Design review of the part built by this model. Coordinates are the model's own, in mm. Face numbers are marked on the shaded views. A direction names the side the tool comes from. Coordinates: 2 decimals unless noted, no trailing zeros. Loops run counter-clockwise (first coordinate to the right, second up) from the corner with the lowest first, then second, coordinate; pieces in that order, holes last. Notation, with made-up numbers: M 69.25,-34.75 L 101.25,-34.75 A23 cw 101.25,-22.75 Z; hole C 36.25,-10.5 d9. An arc over 180 degrees is marked long. Answer as a JSON object with one key per item and string values. Group by question number.
1. Consider section C-C (z = 48.5). State the section outline as (x, y) points.
2. Draft analysis for pull direction X (two halves, no side actions). For the marked faces 4, 5 and 6, state which applies: +X half, -X half, draft (parallel to the pull), parting line (faces both ways), or undercut.
3. Insertion check: pin 1 (1.8 mm diameter, centred on x = 4.22, z = -16.15, fed in from -Y); pin 2 (12 mm diameter, centred on x = 3.5, z = -18.5, fed in from -Y); pin 3 (0.6 mm diameter, centred on y = 1, z = 9, fed in from -X); pin 4 (1 mm diameter, centred on y = 1, z = -19, fed in from +X). Each pin has a flat end and moves straight along its axis. Give the tip position at first contact, or say it passes through.
4. To check wall thickness, follow probe 1 along X at (y, z) = (-17, 42); probe 2 along Y at (x, z) = (22.5, 45.5); probe 3 along Z at (x, y) = (16, -32). State the ranges of each line that lie inside material, in increasing order.
5. Machinability: for the marked faces 1, 2 and 3, which of the approach directions +Z, -Z, +X, -X, +Y, -Y give a long, thin tool a straight path to every point of the face, cutting with its end or side? Answer none if there is none.
6. Consider section A-A (x = -10). State the section outline as (y, z) points, then the cut area to 3 significant figures.
7. Consider section B-B (y = -3). State the section outline as (x, z) points, then the cut area to 3 significant figures.
8. Consider section D-D (z = -1). State the section outline as (x, y) points.
from build123d import *

# Parameters (mm, degrees)
BOSS_EXTRUDE1_DEPTH = 2
SKETCH3_W           = 60.33
SKETCH3_H           = 20
BOSS_EXTRUDE2_DEPTH = 30
SKETCH4_W           = 54.33
SKETCH4_H           = 27
CUT_EXTRUDE1_DEPTH  = 20
SKETCH5_R           = 1.5
CUT_EXTRUDE2_DEPTH  = 2
SKETCH6_W           = 60.33
SKETCH6_H           = 20
BOSS_EXTRUDE3_DEPTH = 5
SKETCH8_W           = 54.33
SKETCH8_H           = 20
CUT_EXTRUDE3_DEPTH  = 3
SKETCH9_W           = 24.33
SKETCH9_H           = 20
BOSS_EXTRUDE4_DEPTH = 2
SKETCH10_R          = 2.5
CUT_EXTRUDE4_DEPTH  = 2


with BuildPart() as part:
    # Sketch2 → Boss-Extrude1 (new body)
    with BuildSketch(Plane(origin=(0, 0, 0), x_dir=(1, 0, 0), z_dir=(0, 1, 0))):
        Polygon((-7.941176471, 23.529411765), (16.388823529, 23.529411765), (16.388823529, -36.470588235), (34.388823529, -36.470588235), (34.388823529, -56.470588235), (-25.941176471, -56.470588235), (-25.941176471, -36.470588235), (-7.941176471, -36.470588235), align=None)
    extrude(amount=BOSS_EXTRUDE1_DEPTH)

    # Sketch3 → Boss-Extrude2 (add)
    with BuildSketch(Plane(origin=(0, 0, 0), x_dir=(-1, 0, 0), z_dir=(0, -1, 0))):
        with Locations((-4.223823529, -46.470588235)):
            Rectangle(SKETCH3_W, SKETCH3_H)
    extrude(amount=BOSS_EXTRUDE2_DEPTH)

    # Sketch4 → Cut-Extrude1 (cut)
    with BuildSketch(Plane(origin=(0, 0, 36.470588235), x_dir=(-1, 0, 0), z_dir=(0, 0, -1))):
        with Locations((-4.223823529, -15)):
            Rectangle(SKETCH4_W, SKETCH4_H)
    extrude(amount=-CUT_EXTRUDE1_DEPTH, mode=Mode.SUBTRACT)

    # Sketch5 → Cut-Extrude2 (cut)
    with BuildSketch(Plane(origin=(0, 0, 0), x_dir=(-1, 0, 0), z_dir=(0, -1, 0))):
        with Locations((-4.223823529, 16.1506031)):
            Circle(SKETCH5_R)
    extrude(amount=-CUT_EXTRUDE2_DEPTH, mode=Mode.SUBTRACT)

    # Sketch6 → Boss-Extrude3 (add)
    with BuildSketch(Plane.XZ.offset(30)):
        with Locations((4.223823529, 46.470588235)):
            Rectangle(SKETCH6_W, SKETCH6_H)
    extrude(amount=BOSS_EXTRUDE3_DEPTH)

    # Sketch8 → Cut-Extrude3 (cut)
    with BuildSketch(Plane(origin=(0, -28.5, 0), x_dir=(1, 0, 0), z_dir=(0, 1, 0))):
        with Locations((4.223823529, -46.470588235)):
            Rectangle(SKETCH8_W, SKETCH8_H)
    extrude(amount=-CUT_EXTRUDE3_DEPTH, mode=Mode.SUBTRACT)

    # Sketch9 → Boss-Extrude4 (add)
    with BuildSketch(Plane(origin=(0, 2, 0), x_dir=(1, 0, 0), z_dir=(0, 1, 0))):
        with Locations((4.223823529, 33.529411765)):
            Rectangle(SKETCH9_W, SKETCH9_H)
    extrude(amount=-BOSS_EXTRUDE4_DEPTH)

    # Sketch10 → Cut-Extrude4 (cut)
    with BuildSketch(Plane(origin=(0, 0, 0), x_dir=(-1, 0, 0), z_dir=(0, -1, 0))):
        with Locations((-4.223823529, 37.893427201)):
            Circle(SKETCH10_R)
    extrude(amount=-CUT_EXTRUDE4_DEPTH, mode=Mode.SUBTRACT)


solid = part.part
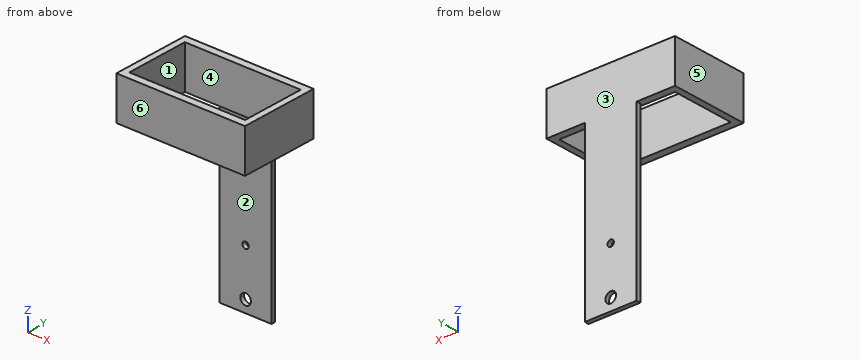
Findings below:
{
 "1": {"outline": "M -25.94,-35 L 34.39,-35 L 34.39,2 L -25.94,2 Z; hole M -22.94,-31.5 L 31.39,-31.5 L 31.39,-1.5 L -22.94,-1.5 Z"},
 "2": {"face 4": "undercut", "face 5": "-X half", "face 6": "draft"},
 "3": {"pin 1": "passes through", "pin 2": "stops at y = 0", "pin 3": "stops at x = -7.94", "pin 4": "stops at x = 16.39"},
 "4": {"probe 1": "x = -25.94 to -22.94, 31.39 to 34.39", "probe 2": "y = -35 to -31.5, -1.5 to 2", "probe 3": "z = 36.47 to 56.47"},
 "5": {"face 1": "+Z, -Z", "face 2": "-Z, +X, -X, -Y", "face 3": "+Z, -Z, +X, -X, +Y"},
 "6": {"outline": "M -35,36.47 L -31.5,36.47 L -31.5,56.47 L -35,56.47 Z; M -1.5,36.47 L 2,36.47 L 2,56.47 L -1.5,56.47 Z", "area": "140 mm^2"},
 "7": {"outline": "M -25.94,36.47 L -22.94,36.47 L -22.94,56.47 L -25.94,56.47 Z; M 31.39,36.47 L 34.39,36.47 L 34.39,56.47 L 31.39,56.47 Z", "area": "120 mm^2"},
 "8": {"outline": "M -7.94,0 L 16.39,0 L 16.39,2 L -7.94,2 Z"}
}
